```python
from build123d import *

# Parameters (mm, degrees)
F1_DEPTH = 3
F2_R     = 1
F3_DEPTH = 3.001


with BuildPart() as f1:
    # F0 (on Front) → F1 (new body)
    with BuildSketch(Plane.XZ):
        with BuildLine():
            ThreePointArc((8.24679, -0.794783), (8.275442, -0.397851), (8.285, 0))
            ThreePointArc((8.285, 0), (8.275442, 0.397851), (8.24679, 0.794783))
            ThreePointArc((8.24679, 0.794783), (8.182998, 1.29606), (8.088765, 1.792514))
            ThreePointArc((8.088765, 1.792514), (7.879503, 2.560206), (7.597562, 3.304282))
            ThreePointArc((7.597562, 3.304282), (7.381989, 3.761311), (7.138955, 4.204348))
            ThreePointArc((7.138955, 4.204348), (6.702706, 4.869801), (6.204631, 5.490335))
            ThreePointArc((6.204631, 5.490335), (5.85838, 5.85838), (5.490335, 6.204631))
            ThreePointArc((5.490335, 6.204631), (4.869801, 6.702706), (4.204348, 7.138955))
            ThreePointArc((4.204348, 7.138955), (3.761311, 7.381989), (3.304282, 7.597562))
            ThreePointArc((3.304282, 7.597562), (2.560206, 7.879503), (1.792514, 8.088765))
            ThreePointArc((1.792514, 8.088765), (1.29606, 8.182998), (0.794783, 8.24679))
            ThreePointArc((0.794783, 8.24679), (0, 8.285), (-0.794783, 8.24679))
            ThreePointArc((-0.794783, 8.24679), (-1.29606, 8.182998), (-1.792514, 8.088765))
            ThreePointArc((-1.792514, 8.088765), (-2.560206, 7.879503), (-3.304282, 7.597562))
            ThreePointArc((-3.304282, 7.597562), (-3.761311, 7.381989), (-4.204348, 7.138955))
            ThreePointArc((-4.204348, 7.138955), (-4.869801, 6.702706), (-5.490335, 6.204631))
            ThreePointArc((-5.490335, 6.204631), (-5.85838, 5.85838), (-6.204631, 5.490335))
            ThreePointArc((-6.204631, 5.490335), (-6.702706, 4.869801), (-7.138955, 4.204348))
            ThreePointArc((-7.138955, 4.204348), (-7.381989, 3.761311), (-7.597562, 3.304282))
            ThreePointArc((-7.597562, 3.304282), (-7.879503, 2.560206), (-8.088765, 1.792514))
            ThreePointArc((-8.088765, 1.792514), (-8.182998, 1.29606), (-8.24679, 0.794783))
            ThreePointArc((-8.24679, 0.794783), (-8.285, 0), (-8.24679, -0.794783))
            ThreePointArc((-8.24679, -0.794783), (-8.182998, -1.29606), (-8.088765, -1.792514))
            ThreePointArc((-8.088765, -1.792514), (-7.879503, -2.560206), (-7.597562, -3.304282))
            ThreePointArc((-7.597562, -3.304282), (-7.381989, -3.761311), (-7.138955, -4.204348))
            ThreePointArc((-7.138955, -4.204348), (-6.702706, -4.869801), (-6.204631, -5.490335))
            ThreePointArc((-6.204631, -5.490335), (-5.85838, -5.85838), (-5.490335, -6.204631))
            ThreePointArc((-5.490335, -6.204631), (-4.869801, -6.702706), (-4.204348, -7.138955))
            ThreePointArc((-4.204348, -7.138955), (-3.761311, -7.381989), (-3.304282, -7.597562))
            ThreePointArc((-3.304282, -7.597562), (-2.560206, -7.879503), (-1.792514, -8.088765))
            ThreePointArc((-1.792514, -8.088765), (-1.29606, -8.182998), (-0.794783, -8.24679))
            ThreePointArc((-0.794783, -8.24679), (0, -8.285), (0.794783, -8.24679))
            ThreePointArc((0.794783, -8.24679), (1.29606, -8.182998), (1.792514, -8.088765))
            ThreePointArc((1.792514, -8.088765), (2.560206, -7.879503), (3.304282, -7.597562))
            ThreePointArc((3.304282, -7.597562), (3.761311, -7.381989), (4.204348, -7.138955))
            ThreePointArc((4.204348, -7.138955), (4.869801, -6.702706), (5.490335, -6.204631))
            ThreePointArc((5.490335, -6.204631), (5.85838, -5.85838), (6.204631, -5.490335))
            ThreePointArc((6.204631, -5.490335), (6.702706, -4.869801), (7.138955, -4.204348))
            ThreePointArc((7.138955, -4.204348), (7.381989, -3.761311), (7.597562, -3.304282))
            ThreePointArc((7.597562, -3.304282), (7.879503, -2.560206), (8.088765, -1.792514))
            ThreePointArc((8.088765, -1.792514), (8.182998, -1.29606), (8.24679, -0.794783))
        make_face()
        with BuildLine():
            ThreePointArc((8.24679, 0.794783), (8.275442, 0.397851), (8.285, 0))
            ThreePointArc((8.285, 0), (8.275442, -0.397851), (8.24679, -0.794783))
            ThreePointArc((8.24679, -0.794783), (9.046963, -0.679903), (9.779182, -0.33737))
            ThreePointArc((9.779182, -0.33737), (9.785, 0), (9.779182, 0.33737))
            ThreePointArc((9.779182, 0.33737), (9.046963, 0.679903), (8.24679, 0.794783))
        make_face()
        with BuildLine():
            ThreePointArc((7.597562, 3.304282), (7.879503, 2.560206), (8.088765, 1.792514))
            ThreePointArc((8.088765, 1.792514), (8.814274, 2.149039), (9.404808, 2.701076))
            ThreePointArc((9.404808, 2.701076), (9.306088, 3.023731), (9.196302, 3.342791))
            ThreePointArc((9.196302, 3.342791), (8.394071, 3.442291), (7.597562, 3.304282))
        make_face()
        with BuildLine():
            ThreePointArc((9.404808, -2.701076), (8.814274, -2.149039), (8.088765, -1.792514))
            ThreePointArc((8.088765, -1.792514), (7.879503, -2.560206), (7.597562, -3.304282))
            ThreePointArc((7.597562, -3.304282), (8.394071, -3.442291), (9.196302, -3.342791))
            ThreePointArc((9.196302, -3.342791), (9.306088, -3.023731), (9.404808, -2.701076))
        make_face()
        with BuildLine():
            ThreePointArc((6.204631, 5.490335), (6.702706, 4.869801), (7.138955, 4.204348))
            ThreePointArc((7.138955, 4.204348), (7.718783, 4.767618), (8.109826, 5.475121))
            ThreePointArc((8.109826, 5.475121), (7.916231, 5.751479), (7.713224, 6.020997))
            ThreePointArc((7.713224, 6.020997), (6.91951, 5.867724), (6.204631, 5.490335))
        make_face()
        with BuildLine():
            ThreePointArc((8.109826, -5.475121), (7.718783, -4.767618), (7.138955, -4.204348))
            ThreePointArc((7.138955, -4.204348), (6.702706, -4.869801), (6.204631, -5.490335))
            ThreePointArc((6.204631, -5.490335), (6.91951, -5.867724), (7.713224, -6.020997))
            ThreePointArc((7.713224, -6.020997), (7.916231, -5.751479), (8.109826, -5.475121))
        make_face()
        with BuildLine():
            ThreePointArc((4.204348, 7.138955), (4.869801, 6.702706), (5.490335, 6.204631))
            ThreePointArc((5.490335, 6.204631), (5.867724, 6.91951), (6.020997, 7.713224))
            ThreePointArc((6.020997, 7.713224), (5.751479, 7.916231), (5.475121, 8.109826))
            ThreePointArc((5.475121, 8.109826), (4.767618, 7.718783), (4.204348, 7.138955))
        make_face()
        with BuildLine():
            ThreePointArc((6.020997, -7.713224), (5.867724, -6.91951), (5.490335, -6.204631))
            ThreePointArc((5.490335, -6.204631), (4.869801, -6.702706), (4.204348, -7.138955))
            ThreePointArc((4.204348, -7.138955), (4.767618, -7.718783), (5.475121, -8.109826))
            ThreePointArc((5.475121, -8.109826), (5.751479, -7.916231), (6.020997, -7.713224))
        make_face()
        with BuildLine():
            ThreePointArc((1.792514, 8.088765), (2.560206, 7.879503), (3.304282, 7.597562))
            ThreePointArc((3.304282, 7.597562), (3.442291, 8.394071), (3.342791, 9.196302))
            ThreePointArc((3.342791, 9.196302), (3.023731, 9.306088), (2.701076, 9.404808))
            ThreePointArc((2.701076, 9.404808), (2.149039, 8.814274), (1.792514, 8.088765))
        make_face()
        with BuildLine():
            ThreePointArc((3.342791, -9.196302), (3.442291, -8.394071), (3.304282, -7.597562))
            ThreePointArc((3.304282, -7.597562), (2.560206, -7.879503), (1.792514, -8.088765))
            ThreePointArc((1.792514, -8.088765), (2.149039, -8.814274), (2.701076, -9.404808))
            ThreePointArc((2.701076, -9.404808), (3.023731, -9.306088), (3.342791, -9.196302))
        make_face()
        with BuildLine():
            ThreePointArc((-0.794783, 8.24679), (0, 8.285), (0.794783, 8.24679))
            ThreePointArc((0.794783, 8.24679), (0.679903, 9.046963), (0.33737, 9.779182))
            ThreePointArc((0.33737, 9.779182), (0, 9.785), (-0.33737, 9.779182))
            ThreePointArc((-0.33737, 9.779182), (-0.679903, 9.046963), (-0.794783, 8.24679))
        make_face()
        with BuildLine():
            ThreePointArc((0.33737, -9.779182), (0.679903, -9.046963), (0.794783, -8.24679))
            ThreePointArc((0.794783, -8.24679), (0, -8.285), (-0.794783, -8.24679))
            ThreePointArc((-0.794783, -8.24679), (-0.679903, -9.046963), (-0.33737, -9.779182))
            ThreePointArc((-0.33737, -9.779182), (0, -9.785), (0.33737, -9.779182))
        make_face()
        with BuildLine():
            ThreePointArc((-3.304282, 7.597562), (-2.560206, 7.879503), (-1.792514, 8.088765))
            ThreePointArc((-1.792514, 8.088765), (-2.149039, 8.814274), (-2.701076, 9.404808))
            ThreePointArc((-2.701076, 9.404808), (-3.023731, 9.306088), (-3.342791, 9.196302))
            ThreePointArc((-3.342791, 9.196302), (-3.442291, 8.394071), (-3.304282, 7.597562))
        make_face()
        with BuildLine():
            ThreePointArc((-2.701076, -9.404808), (-2.149039, -8.814274), (-1.792514, -8.088765))
            ThreePointArc((-1.792514, -8.088765), (-2.560206, -7.879503), (-3.304282, -7.597562))
            ThreePointArc((-3.304282, -7.597562), (-3.442291, -8.394071), (-3.342791, -9.196302))
            ThreePointArc((-3.342791, -9.196302), (-3.023731, -9.306088), (-2.701076, -9.404808))
        make_face()
        with BuildLine():
            ThreePointArc((-5.490335, 6.204631), (-4.869801, 6.702706), (-4.204348, 7.138955))
            ThreePointArc((-4.204348, 7.138955), (-4.767618, 7.718783), (-5.475121, 8.109826))
            ThreePointArc((-5.475121, 8.109826), (-5.751479, 7.916231), (-6.020997, 7.713224))
            ThreePointArc((-6.020997, 7.713224), (-5.867724, 6.91951), (-5.490335, 6.204631))
        make_face()
        with BuildLine():
            ThreePointArc((-5.475121, -8.109826), (-4.767618, -7.718783), (-4.204348, -7.138955))
            ThreePointArc((-4.204348, -7.138955), (-4.869801, -6.702706), (-5.490335, -6.204631))
            ThreePointArc((-5.490335, -6.204631), (-5.867724, -6.91951), (-6.020997, -7.713224))
            ThreePointArc((-6.020997, -7.713224), (-5.751479, -7.916231), (-5.475121, -8.109826))
        make_face()
        with BuildLine():
            ThreePointArc((-7.138955, 4.204348), (-6.702706, 4.869801), (-6.204631, 5.490335))
            ThreePointArc((-6.204631, 5.490335), (-6.91951, 5.867724), (-7.713224, 6.020997))
            ThreePointArc((-7.713224, 6.020997), (-7.916231, 5.751479), (-8.109826, 5.475121))
            ThreePointArc((-8.109826, 5.475121), (-7.718783, 4.767618), (-7.138955, 4.204348))
        make_face()
        with BuildLine():
            ThreePointArc((-7.713224, -6.020997), (-6.91951, -5.867724), (-6.204631, -5.490335))
            ThreePointArc((-6.204631, -5.490335), (-6.702706, -4.869801), (-7.138955, -4.204348))
            ThreePointArc((-7.138955, -4.204348), (-7.718783, -4.767618), (-8.109826, -5.475121))
            ThreePointArc((-8.109826, -5.475121), (-7.916231, -5.751479), (-7.713224, -6.020997))
        make_face()
        with BuildLine():
            ThreePointArc((-8.088765, 1.792514), (-7.879503, 2.560206), (-7.597562, 3.304282))
            ThreePointArc((-7.597562, 3.304282), (-8.394071, 3.442291), (-9.196302, 3.342791))
            ThreePointArc((-9.196302, 3.342791), (-9.306088, 3.023731), (-9.404808, 2.701076))
            ThreePointArc((-9.404808, 2.701076), (-8.814274, 2.149039), (-8.088765, 1.792514))
        make_face()
        with BuildLine():
            ThreePointArc((-9.196302, -3.342791), (-8.394071, -3.442291), (-7.597562, -3.304282))
            ThreePointArc((-7.597562, -3.304282), (-7.879503, -2.560206), (-8.088765, -1.792514))
            ThreePointArc((-8.088765, -1.792514), (-8.814274, -2.149039), (-9.404808, -2.701076))
            ThreePointArc((-9.404808, -2.701076), (-9.306088, -3.023731), (-9.196302, -3.342791))
        make_face()
        with BuildLine():
            ThreePointArc((-8.24679, -0.794783), (-8.285, 0), (-8.24679, 0.794783))
            ThreePointArc((-8.24679, 0.794783), (-9.046963, 0.679903), (-9.779182, 0.33737))
            ThreePointArc((-9.779182, 0.33737), (-9.785, 0), (-9.779182, -0.33737))
            ThreePointArc((-9.779182, -0.33737), (-9.046963, -0.679903), (-8.24679, -0.794783))
        make_face()
    extrude(amount=F1_DEPTH)

    # F2 (on face) → F3 (cut, through all)
    with BuildSketch(Plane(origin=(0, 0, 0), x_dir=(-1, 0, 0), z_dir=(0, 1, 0))):
        Circle(F2_R)
    extrude(amount=-F3_DEPTH, mode=Mode.SUBTRACT)


with BuildPart() as f4_1:
    # F4: copy of F1
    add(f1.part)


solid = f1.part
```
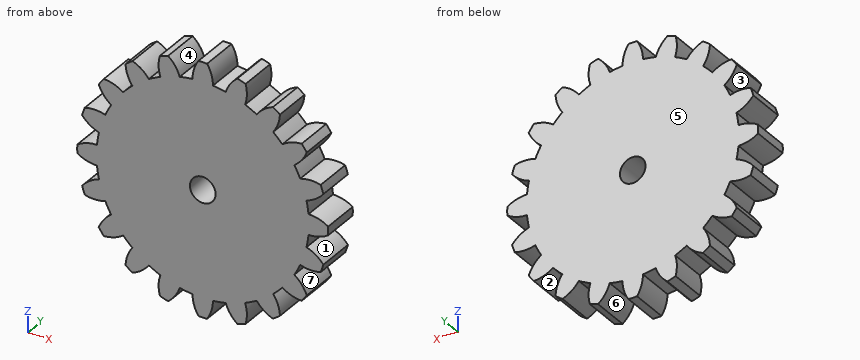
Can you work these out from the model? Positions are in its coordinate system, mm. Face numbers are marked on the shaded views. A direction names the side the tool comes from. Coordinates: 2 decimals unless noted, no trailing zeros. Order: outer loops, then holes, each group sorted by start corner. A loop starts at its lowest first (then second) coordinate and runs counter-clockwise, first axis right, second up. Notation, with made-up numbers: (35.25, -7) -> (76.25, -7) arc R21 cw to (76.25, 19) -> close; hole circle Ø7 at (-39, 51.5). An arc over 180 degrees is marked (long way). Write each question's results on one line, items separated by ' | '.
Item 1: I'm going to push a flat-ended pin straight in: pin 1 Ø1.5 at (x, y) = (-4.5, -0.5) entering from +Z. Where does the tip first touch, or does it pass through?
Results are:
pin 1: z = 8.01
Item 2: I want a section at C-C, the plane z = -8.5. Write out the boundary of the cut face in (x, y).
Results are:
outline: (-3.44, -3) -> (-1.96, -3) -> (-1.96, 0) -> (-3.44, 0) -> close; (-0.78, -3) -> (0.78, -3) -> (0.78, 0) -> (-0.78, 0) -> close; (1.96, -3) -> (3.44, -3) -> (3.44, 0) -> (1.96, 0) -> close
Item 3: Which directions (+Z, -Z, +X, -X, +Y, -Y) give clear straight access to the entire face, cutting with the end or side of a thin tool? Please do the marked faces 1, 2 and 3.
Results are:
face 1: +X, +Y, -Y | face 2: -Z, +Y, -Y | face 3: -X, +Y, -Y
Item 4: I want a section at A-A, the plane x = 0. Write out the boundary of the cut face in (y, z) (3 decimals), then the cut area to 3 significant figures.
Results are:
outline: (-3, -9.785) -> (0, -9.785) -> (0, -1) -> (-3, -1) -> close; (-3, 1) -> (0, 1) -> (0, 9.785) -> (-3, 9.785) -> close | area: 52.7 mm²
Item 5: If I drill on line 1 along Z through (x, y) = (0, -0.65) (3 decimals); line 2 along X through (y, z) = (-2.5, -8.5), over which ranges is the centre line in solid material (lowest first)?
Results are:
line 1: -9.785 to -1, 1 to 9.785 | line 2: -3.44 to -1.96, -0.78 to 0.78, 1.96 to 3.44
Item 6: If we mould it in two halves opening along X, with no side actions, what happens to the marked faces 4, 5, 6 and 7? For each: +X half, -X half, draft (parallel to the pull), parting line (faces both ways), or undercut.
Results are:
face 4: undercut | face 5: draft | face 6: undercut | face 7: +X half
Item 7: I want a section at B-B, the plane z = 0. Write out the boundary of the cut face in (x, y) (3 decimals).
Results are:
outline: (-9.785, -3) -> (-1, -3) -> (-1, 0) -> (-9.785, 0) -> close; (1, -3) -> (9.785, -3) -> (9.785, 0) -> (1, 0) -> close
Item 8: I want a section at D-D, the plane x = 4.5. Write out the boundary of the cut face in (y, z), then the cut area to 3 significant figures.
Results are:
outline: (-3, -7.49) -> (0, -7.49) -> (0, 7.49) -> (-3, 7.49) -> close | area: 44.9 mm²
